The figure shows three views and two pictorial views of one solid part (mm, origin at its lowest corner). Answer the questions. Round coordinates to 2 decimals unless told otherwise and drop trailing zeros. Order: outer loops, then holes, each group sorted by start corner. A loop starts at its lowest first (then second) coordinate and runs counter-clockwise, first axis right, second up. Notation, with made-up numbers: (67.25, 73.5) - (80.25, 73.5) arc R26 ccw to (80.25, 94.5) - close; hole circle Ø9 at (30, -23). An arc over 180 degrees is marked (long way). Use CSV: the item, a comma, the result in double quotes.
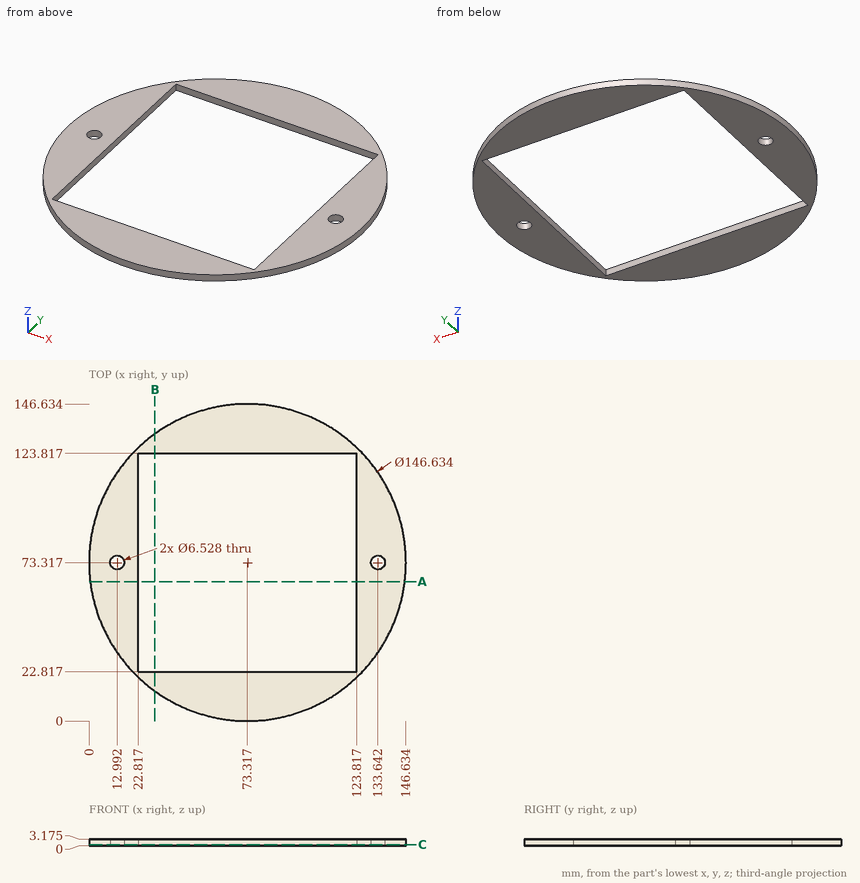
(1) Find the intervals of material crossed by L1, parallel to X at y = 72.5, z = 0.7 (1 decimal); L2, parallel to X at y = 118, z = 0.3 (1 decimal); L3, parallel to Y at x = 62, z = 2.15 (1 decimal), in increasing order. Write a range as from..to.
Findings below:
L1,"x = 0..9.8, 16.2..22.8, 123.8..130.5, 136.8..146.6"
L2,"x = 15.2..22.8, 123.8..131.4"
L3,"y = 0.9..22.8, 123.8..145.8"
(2) Find section A-A (y = 64.5). Determine the outline of the cut face in (x, z) (1 decimal).
Findings below:
outline,"(0.5, 0) - (22.8, 0) - (22.8, 3.2) - (0.5, 3.2) - close; (123.8, 0) - (146.1, 0) - (146.1, 3.2) - (123.8, 3.2) - close"
(3) Find section C-C (z = 0.6). Determine the outline of the cut face in (x, y).
Findings below:
outline,"circle Ø146.63 at (73.32, 73.32); hole circle Ø6.53 at (12.99, 73.32); hole (22.82, 22.82) - (123.82, 22.82) - (123.82, 123.82) - (22.82, 123.82) - close; hole circle Ø6.53 at (133.64, 73.32)"
(4) Find section B-B (x = 30.5). Determine the outline of the cut face in (y, z) (1 decimal).
Findings below:
outline,"(13.8, 0) - (22.8, 0) - (22.8, 3.2) - (13.8, 3.2) - close; (123.8, 0) - (132.8, 0) - (132.8, 3.2) - (123.8, 3.2) - close"
(5) Each of these flat-tipped pins is pushed along its axis until it touches: pin 1 (1 mm diameter, centred on x = 95.5, z = 1, fed in from -Y); pin 2 (1 mm diameter, centred on y = 57, z = 1, fed in from +X). Where does it stop, or does it pass through?
Findings below:
pin 1,"stops at y = 3.28"
pin 2,"stops at x = 144.91"
